from build123d import *

# Parameters (mm, degrees)
F_6_6_6_6_DIAMETER_HOLE1_D = 6.6


with BuildPart() as part:
    # Sketch1 → Revolve1 (revolve)
    with BuildSketch(Plane.XY, mode=Mode.PRIVATE) as revolve1_sk:
        Polygon((15, 38), (15, 0), (32.5, 0), (32.5, 9.5), (19, 9.5), (19, 38), align=None)
    revolve(revolve1_sk.sketch.rotate(Axis((0, 0, 0), (0, 1, 0)), 90), axis=Axis((0, 0, 0), (0, 1, 0)))

    # 6.6 _6.6_ Diameter Hole1 (through all)
    with Locations(Plane(origin=(0, 9.5, 0), x_dir=(1, 0, 0), z_dir=(0, 1, 0))):
        with Locations((0, 26), (0, -26), (26, 0), (-26, 0)):
            Hole(F_6_6_6_6_DIAMETER_HOLE1_D / 2)


solid = part.part
CAD build for the part. Positions are in the model's coordinates, mm. A direction names the side the tool comes from. Coordinates: 2 decimals unless noted, no trailing zeros. Write each loop counter-clockwise with the first axis right and the second up, starting at its lowest first coordinate (ties: lowest second). Pieces come first, ordered by that corner, then holes. Notation, with made-up numbers: M 17.5,-21.75 L 75.5,-21.75 A17 ccw 75.5,-8.75 Z; hole C 6.25,10 d1. An arc over 180 degrees is marked long. Answer as a JSON object with one key per item and string values. Group by question number.
1) Wall check: line 1 (X direction, y = 18, z = 0); line 2 (Y direction, x = 5.5, z = 24.5); line 3 (Z direction, x = -13, y = 6). Give the ranges that are in metal, low to high. Write a range as from..to.
2) Mould opens along Z. For faces 3 (the face through (-9.76, 4.82, -31)), 4 (the face through (-6, 38, -14)), 5 (the face through (22.95, 4.68, 1.26)) say: +Z half, -Z half, draft (parallel to the pull), parting line (faces both ways), or undercut.
3) Saw through at D-D (x = 0). Write the cut outline in (y, z), plus the area to 3 significant figures.
4) Saw through at A-A (z = 26). Write the cut outline in (x, y).
5) Saw through at C-C (z = 0). Write the cut outline in (x, y).
6) Pin check, flat tips, straight feed: pin 1 Ø8.5 at (x, z) = (-26, 0) entering from +Y; pin 2 Ø4 at (y, z) = (21.5, -18.5) entering from -X; pin 3 Ø1.5 at (y, z) = (12.5, -13.5) entering from +X. Stop position of each tip, or through.
7) Saw through at B-B (x = -26). Write the cut outline in (y, z).
8) Tool access for faces 1 (the face through (0.72, 4.68, -22.78)), 2 (the face through (18.548, 23.95, 4.119)): list every direction of +Z, -Z, +X, -X, +Y, -Y with a clear straight run to the whole face (end or side of a thin tool).
Values follow:
{
 "1": {"line 1": "x = -19..-15, 15..19", "line 2": "y = 0..9.5", "line 3": "z = -29.79..-7.48, 7.48..29.79"},
 "2": {"face 3": "parting line", "face 4": "draft", "face 5": "undercut"},
 "3": {"outline": "M 0,-32.5 L 9.5,-32.5 L 9.5,-29.3 L 0,-29.3 Z; M 0,-22.7 L 9.5,-22.7 L 9.5,-19 L 38,-19 L 38,-15 L 0,-15 Z; M 0,15 L 38,15 L 38,19 L 9.5,19 L 9.5,22.7 L 0,22.7 Z; M 0,29.3 L 9.5,29.3 L 9.5,32.5 L 0,32.5 Z", "area": "435 mm2"},
 "4": {"outline": "M -19.5,0 L -3.3,0 L -3.3,9.5 L -19.5,9.5 Z; M 3.3,0 L 19.5,0 L 19.5,9.5 L 3.3,9.5 Z"},
 "5": {"outline": "M -32.5,0 L -29.3,0 L -29.3,9.5 L -32.5,9.5 Z; M -22.7,0 L -15,0 L -15,38 L -19,38 L -19,9.5 L -22.7,9.5 Z; M 15,0 L 22.7,0 L 22.7,9.5 L 19,9.5 L 19,38 L 15,38 Z; M 29.3,0 L 32.5,0 L 32.5,9.5 L 29.3,9.5 Z"},
 "6": {"pin 1": "stops at y = 9.5", "pin 2": "stops at x = -9.42", "pin 3": "stops at x = 14.09"},
 "7": {"outline": "M 0,-19.5 L 9.5,-19.5 L 9.5,-3.3 L 0,-3.3 Z; M 0,3.3 L 9.5,3.3 L 9.5,19.5 L 0,19.5 Z"},
 "8": {"face 1": "+Y, -Y", "face 2": "+Y"}
}
